Here's how the part is built. I have some questions about the finished solid (model axes, mm). Face numbers are marked on the shaded views. A direction names the side the tool comes from. Round coordinates to 2 decimals unless told otherwise and drop trailing zeros. Order: outer loops, then holes, each group sorted by start corner. A loop starts at its lowest first (then second) coordinate and runs counter-clockwise, first axis right, second up. Notation, with made-up numbers: (-39, 29.5) - (18, 29.5) arc R28 ccw to (18, 48.5) - close; hole circle Ø6 at (-19.75, 74.5). An arc over 180 degrees is marked (long way). Answer as a JSON object with one key per item and string values.
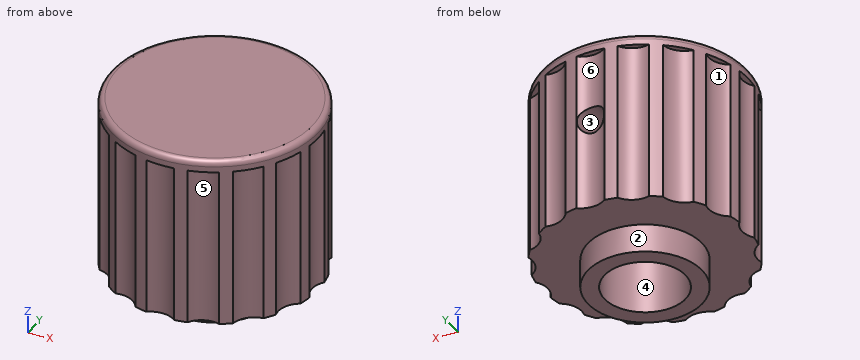
```python
from build123d import *

# Parameters (mm, degrees)
F2_R      = 3.55
F3_DEPTH  = 16.5
F5_DEPTH  = 9
F6_R      = 0.5
F7_R      = 1.2
F8_DEPTH  = 10
F9_R      = 2
F10_DEPTH = 14


with BuildPart() as f1:
    # F0 (on Front) → F1 (revolve)
    with BuildSketch(Plane.XZ):
        Polygon((-5, 0), (0, 0), (0, 17.5), (-9, 17.5), (-9, 2.5), (-5, 2.5), align=None)
    revolve(axis=Axis((0, 0, -3.667768), (0, 0, -1)))

    # F2 (on face) → F3 (cut)
    with BuildSketch(Plane(origin=(0, 0, 0), x_dir=(1, 0, 0), z_dir=(0, 0, -1))):
        Circle(F2_R)
    extrude(amount=-F3_DEPTH, mode=Mode.SUBTRACT)

    # F4 (on face) → F5 (join)
    with BuildSketch(Plane(origin=(0, 0, 16.5), x_dir=(1, 0, 0), z_dir=(0, 0, -1))):
        with BuildLine():
            Line((3.207453, -1.521429), (-3.207453, -1.521429))
            ThreePointArc((-3.207453, -1.521429), (0, -3.55), (3.207453, -1.521429))
        make_face()
    extrude(amount=F5_DEPTH)

    # F6
    f6_edges = [f1.edges().sort_by_distance(p)[0] for p in [
        (9, 0, 17.5),
    ]]
    fillet(f6_edges, radius=F6_R)

    # F7 (on face) → F8 (cut)
    with BuildSketch(Plane.XZ.offset(-1.521429)):
        with Locations((0, 10.5)):
            Circle(F7_R)
    extrude(amount=-F8_DEPTH, mode=Mode.SUBTRACT)

    # F9 (on face) → F10 (cut)
    with BuildSketch(Plane(origin=(0, 0, 2.5), x_dir=(1, 0, 0), z_dir=(0, 0, -1))):
        with Locations((-10.5, 0)):
            Circle(F9_R)
        with Locations((-9.700735, -4.018176)):
            Circle(F9_R)
        with Locations((-7.424621, -7.424621)):
            Circle(F9_R)
        with Locations((-4.018176, -9.700735)):
            Circle(F9_R)
        with Locations((0, -10.5)):
            Circle(F9_R)
        with Locations((4.018176, -9.700735)):
            Circle(F9_R)
        with Locations((7.424621, -7.424621)):
            Circle(F9_R)
        with Locations((9.700735, -4.018176)):
            Circle(F9_R)
        with Locations((10.5, 0)):
            Circle(F9_R)
        with Locations((9.700735, 4.018176)):
            Circle(F9_R)
        with Locations((7.424621, 7.424621)):
            Circle(F9_R)
        with Locations((4.018176, 9.700735)):
            Circle(F9_R)
        with Locations((0, 10.5)):
            Circle(F9_R)
        with Locations((-4.018176, 9.700735)):
            Circle(F9_R)
        with Locations((-7.424621, 7.424621)):
            Circle(F9_R)
        with Locations((-9.700735, 4.018176)):
            Circle(F9_R)
    extrude(amount=-F10_DEPTH, mode=Mode.SUBTRACT)


solid = f1.part
```
1. For the marked faces 4, 5 and 6, which set-ups out of +Z, -Z, +X, -X, +Y, -Y let a thin tool reach every point of the face, with its end or its side?
Responses:
{"face 4": "-Z", "face 5": "-Z, -Y", "face 6": "-Z, +Y"}
2. If I drill on L1, parallel to Z at x = 0, y = 5.5; L2, parallel to Z at x = 8.25, y = -0.5; L3, parallel to Z at x = -2.5, y = 0.5, over which ranges is the centre line in solid material (lowest first)? Write a range as [from, to].
Responses:
{"L1": "[2.5, 9.3], [11.7, 17.5]", "L2": "[2.5, 17.5]", "L3": "[16.5, 17.5]"}
3. Thinking about a two-plate mould opening in X: for the marked faces 1, 2 and 3, which applies, pulls with the +X half, pulls with the -X half, needs draft (parallel to the pull), parting line crosses it, or undercut?
Responses:
{"face 1": "pulls with the -X half", "face 2": "parting line crosses it", "face 3": "undercut"}
4. Imagine slicing it at B-B (y = 0). List the corners of the cut face in (x, z) for me.
Responses:
{"outline": "(-9, 16.5) - (-8.5, 16.5) - (-8.5, 2.5) - (-5, 2.5) - (-5, 0) - (-3.55, 0) - (-3.55, 16.5) - (3.55, 16.5) - (3.55, 0) - (5, 0) - (5, 2.5) - (8.5, 2.5) - (8.5, 16.5) - (9, 16.5) - (9, 17) arc R0.5 ccw to (8.5, 17.5) - (-8.5, 17.5) arc R0.5 ccw to (-9, 17) - close"}
5. For P1, Ø1.9, axis at x = 1.5, z = 12, coming from the -Y side; P2, Ø1.9, axis at x = 0, z = 10.5, coming from the -Y side; P3, Ø2.5, axis at x = -1, y = -1, coming from the -Z side, each with a flat end and sliding along its axis, tell me the tip position at first contact or that it passes through.
Responses:
{"P1": "y = -8.92", "P2": "y = -8.74", "P3": "z = 16.5"}
6. Imagine slicing it at A-A (x = 0). List the corners of the cut face in (y, z) for me, plus the area to 3 significant figures.
Responses:
{"outline": "(-9, 16.5) - (-8.5, 16.5) - (-8.5, 2.5) - (-5, 2.5) - (-5, 0) - (-3.55, 0) - (-3.55, 16.5) - (1.52, 16.5) - (1.52, 11.7) - (8.5, 11.7) - (8.5, 16.5) - (9, 16.5) - (9, 17) arc R0.5 ccw to (8.5, 17.5) - (-8.5, 17.5) arc R0.5 ccw to (-9, 17) - close; (1.52, 7.5) - (3.55, 7.5) - (3.55, 0) - (5, 0) - (5, 2.5) - (8.5, 2.5) - (8.5, 9.3) - (1.52, 9.3) - close", "area": "165 mm2"}
